from build123d import *
from build123d.topology import SkipClean

# Parameters (mm, degrees)
SKETCH1_R           = 4.4
BOSS_EXTRUDE1_DEPTH = 6
SKETCH2_R           = 2.4
BOSS_EXTRUDE2_DEPTH = 2
BOSS_EXTRUDE3_DEPTH = 5
BOSS_EXTRUDE4_START = 2
SKETCH4_W           = 2.9
SKETCH4_H           = 2.9
BOSS_EXTRUDE4_DEPTH = 2


with BuildPart() as part:
    # Sketch1 → Boss-Extrude1 (new body)
    with BuildSketch(Plane(origin=(0, 0, 0), x_dir=(1, 0, 0), z_dir=(0, 1, 0))):
        with Locations(Location((0, 0, 0), (0, 0, 270))):
            Circle(SKETCH1_R)
    extrude(amount=BOSS_EXTRUDE1_DEPTH)

    # Sketch2 → Boss-Extrude2 (add)
    with BuildSketch(Plane(origin=(0, 6, 0), x_dir=(1, 0, 0), z_dir=(0, 1, 0))):
        with Locations(Location((0, 0, 0), (0, 0, 270))):
            Circle(SKETCH2_R)
    extrude(amount=BOSS_EXTRUDE2_DEPTH)

    # Sketch3 → Boss-Extrude3 (add)
    with BuildSketch(Plane(origin=(0, 8, 0), x_dir=(1, 0, 0), z_dir=(0, 1, 0))):
        with BuildLine():
            Line((-1.5, 1.8734994), (-1.5, -1.8734994))
            ThreePointArc((-1.5, -1.8734994), (0, -2.4), (1.5, -1.8734994))
            Line((1.5, -1.8734994), (1.5, 1.8734994))
            ThreePointArc((1.5, 1.8734994), (0, 2.4), (-1.5, 1.8734994))
        make_face()
    extrude(amount=BOSS_EXTRUDE3_DEPTH)

    # Sketch4 → Boss-Extrude4 (add)
    with SkipClean():  # the faces are left unmerged after this step: merging them gives an invalid solid
        with BuildSketch(Plane.XZ.offset(BOSS_EXTRUDE4_START)):
            with BuildLine():
                Line((1.45, -1.45), (-1.45, -1.45))
                Line((-1.45, -1.45), (-1.45, -4.154214727))
                ThreePointArc((-1.45, -4.154214727), (0, -4.4), (1.45, -4.154214727))
                Line((1.45, -4.154214727), (1.45, -1.45))
            make_face()
            Rectangle(SKETCH4_W, SKETCH4_H)
            with BuildLine():
                Line((4.154214727, 1.45), (1.45, 1.45))
                Line((1.45, 1.45), (1.45, -1.45))
                Line((1.45, -1.45), (4.154214727, -1.45))
                ThreePointArc((4.154214727, -1.45), (4.338118532, -0.735341825), (4.4, 0))
                ThreePointArc((4.4, 0), (4.338118532, 0.735341825), (4.154214727, 1.45))
            make_face()
            with BuildLine():
                Line((-1.45, 1.45), (-4.154214727, 1.45))
                ThreePointArc((-4.154214727, 1.45), (-4.4, 0), (-4.154214727, -1.45))
                Line((-4.154214727, -1.45), (-1.45, -1.45))
                Line((-1.45, -1.45), (-1.45, 1.45))
            make_face()
            with BuildLine():
                Line((-1.45, 4.154214727), (-1.45, 1.45))
                Line((-1.45, 1.45), (1.45, 1.45))
                Line((1.45, 1.45), (1.45, 4.154214727))
                ThreePointArc((1.45, 4.154214727), (0, 4.4), (-1.45, 4.154214727))
            make_face()
        extrude(amount=-BOSS_EXTRUDE4_DEPTH)


solid = part.part
Part model, mm, in its own coordinate system. A direction names the side the tool comes from. Round coordinates to 2 decimals unless told otherwise and drop trailing zeros. Write each loop counter-clockwise with the first axis right and the second up, starting at its lowest first coordinate (ties: lowest second). Pieces come first, ordered by that corner, then holes. Notation, with made-up numbers: M 50,39.5 L 75,39.5 A24 cw 75,76.5 Z; hole C 73.25,6.25 d3. An arc over 180 degrees is marked long. Return JSON: item names as keys, results as strings. Group by question number.
(1) Saw through at D-D on x = 2. Write the cut outline in (y, z), then the cut area to 3 significant figures.
(2) Pin check, flat tips, straight feed: pin 1 Ø1.1 at (y, z) = (9.5, 0.5) entering from +X; pin 2 Ø1.6 at (x, y) = (-2.5, -0.5) entering from +Z; pin 3 Ø1 at (x, y) = (-1.5, 2) entering from -Z. Stop position of each tip, or through.
(3) Saw through at B-B on z = 1. Write the cut outline in (x, y).
(4) Which spindle directions (+Z, -Z, +X, -X, +Y, -Y) get a long thin tool onto all of the face, cutting with end or side? Do faces 1 (the face through (3, -1, 1.45)), 2 (the face through (-3, -1, -1.45)), 3 (the face through (2, 8, 0)), 4 (the face through (-2, 8, 0)), 5 (the face through (-1.45, -1, 3)). Say none if no direction does.
(5) Saw through at A-A on x = -3.5. Write the cut outline in (y, z), then the cut area to 3 significant figures.
(6) Saw through at C-C on y = 5.75. Write the cut outline in (x, z), then the cut area to 3 significant figures.
(7) Drill centre lines: probe 1 along X at (y, z) = (11.5, -1.75); probe 2 along Y at (x, z) = (3.5, 2); probe 3 along Y at (x, z) = (1.75, -0.75). Where is each one in solid material? Low to high.
Returned:
{
 "1": {"outline": "M -2,-1.45 L 0,-1.45 L 0,-3.92 L 6,-3.92 L 6,-1.33 L 8,-1.33 L 8,1.33 L 6,1.33 L 6,3.92 L 0,3.92 L 0,1.45 L -2,1.45 Z", "area": "58.1 mm²"},
 "2": {"pin 1": "x = 1.5", "pin 2": "z = 3.98", "pin 3": "z = -4.28"},
 "3": {"outline": "M -4.28,-2 L 4.28,-2 L 4.28,6 L 2.18,6 L 2.18,8 L 1.5,8 L 1.5,13 L -1.5,13 L -1.5,8 L -2.18,8 L -2.18,6 L -4.28,6 Z"},
 "4": {"face 1": "+Z, +X, -Y", "face 2": "-Z, -X, -Y", "face 3": "+Z, -Z, +X, +Y", "face 4": "+Z, -Z, -X, +Y", "face 5": "+Z, -X, -Y"},
 "5": {"outline": "M -2,-1.45 L 0,-1.45 L 0,-2.67 L 6,-2.67 L 6,2.67 L 0,2.67 L 0,1.45 L -2,1.45 Z", "area": "37.8 mm²"},
 "6": {"outline": "C 0,0 d8.8", "area": "60.8 mm²"},
 "7": {"probe 1": "-1.5 to 1.5", "probe 2": "0 to 6", "probe 3": "-2 to 8"}
}
